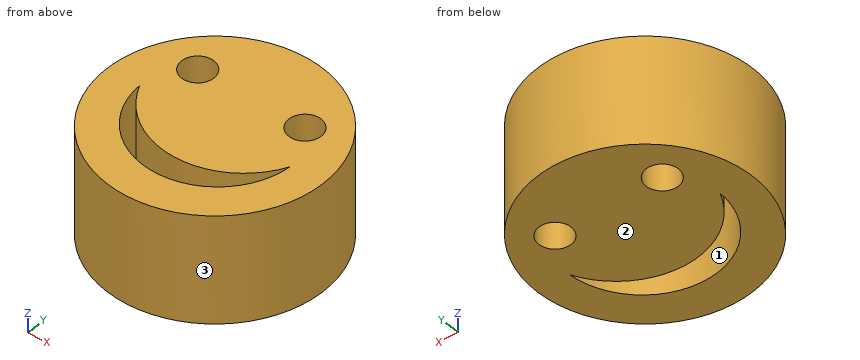
```python
from build123d import *

# Parameters (mm, degrees)
F0_R     = 25.4
F0_R_2   = 3.81
F1_DEPTH = 25.4


with BuildPart() as f1:
    # F0 (on Top) → F1 (new body)
    with BuildSketch(Plane.XY):
        Circle(F0_R)
        with BuildLine():
            ThreePointArc((17.78, 0), (0, -17.018), (-17.78, 0))
            ThreePointArc((-17.78, 0), (0, -11.43), (17.78, 0))
        make_face(mode=Mode.SUBTRACT)
        with Locations((-12.7, 10.16)):
            Circle(F0_R_2, mode=Mode.SUBTRACT)
        with Locations((12.7, 10.16)):
            Circle(F0_R_2, mode=Mode.SUBTRACT)
    extrude(amount=F1_DEPTH)


solid = f1.part
```
Geometry: final body of the model. Coordinates: model frame, mm. Face numbers are marked on the shaded views. Round coordinates to 2 decimals unless told otherwise and drop trailing zeros. Write each loop counter-clockwise with the first axis right and the second up, starting at its lowest first coordinate (ties: lowest second). Pieces come first, ordered by that corner, then holes. Notation, with made-up numbers: (45.5, -32.5) -> (59.5, -32.5) arc R17 cw to (59.5, -7.5) -> close; hole circle Ø11 at (56, -28). An arc over 180 degrees is marked (long way). Use CSV: the item, a comma, the result in double quotes. Start each with the question number.
Q1. First-contact query: pin 1 Ø1 at (x, z) = (-11.5, 19.5) entering from +Y; pin 2 Ø5 at (y, z) = (-19.5, 20) entering from +X; pin 3 Ø6 at (y, z) = (19, 9) entering from +X. Flat tips, straight axial feed; report the tip coordinate or a pass-through.
Q2. Section B-B (x = 12.7). Return loops of the section in (y, z), plus the area to 3 significant figures.
Q3. Section A-A (y = -15). Return loops of the section in (x, z).
Q4. Section C-C (z = 19). Return loops of the section in (x, y).
Q5. Line query: L1, parallel to Y at x = -12.7, z = 7; L2, parallel to Y at x = 11, z = 4.5; L3, parallel to X at y = 11, z = 5.25. Output: solid intervals per line, ascending.
Q6. Section D-D (y = 10.16). Return loops of the section in (x, z), plus the area to 4 significant figures.
Q7. Pull-direction query (X, two-part tool) for the marked faces 1, 2 and 3; classes: pulls with the +X half, pulls with the -X half, needs draft (parallel to the pull), parting line crosses it, or undercut.
Result sheet:
1,pin 1,"y = 22.89"
1,pin 2,"x = 18.87"
1,pin 3,"x = 19.73"
2,outline,"(-22, 0) -> (-11.69, 0) -> (-11.69, 25.4) -> (-22, 25.4) -> close; (-6.74, 0) -> (6.35, 0) -> (6.35, 25.4) -> (-6.74, 25.4) -> close; (13.97, 0) -> (22, 0) -> (22, 25.4) -> (13.97, 25.4) -> close"
2,area,"798 mm²"
3,outline,"(-20.5, 0) -> (-8.23, 0) -> (-8.23, 25.4) -> (-20.5, 25.4) -> close; (8.23, 0) -> (20.5, 0) -> (20.5, 25.4) -> (8.23, 25.4) -> close"
4,outline,"circle Ø50.8 at (0, 0); hole (-17.78, 0) arc R17.8 ccw to (17.78, 0) arc R19.54 cw to start; hole circle Ø7.62 at (-12.7, 10.16); hole circle Ø7.62 at (12.7, 10.16)"
5,L1,"-22 to -11.69, -6.74 to 6.35, 13.97 to 22"
5,L2,"-22.89 to -13.21, -8.04 to 6.75, 13.57 to 22.89"
5,L3,"-22.89 to -16.42, -8.98 to 8.98, 16.42 to 22.89"
6,outline,"(-23.28, 0) -> (-16.51, 0) -> (-16.51, 25.4) -> (-23.28, 25.4) -> close; (-8.89, 0) -> (8.89, 0) -> (8.89, 25.4) -> (-8.89, 25.4) -> close; (16.51, 0) -> (23.28, 0) -> (23.28, 25.4) -> (16.51, 25.4) -> close"
6,area,"795.5 mm²"
7,face 1,"undercut"
7,face 2,"needs draft"
7,face 3,"parting line crosses it"
